Verification items for this drawing (mm, ordinates from the low corner). A direction names the side the tool comes from. Coordinates: 2 decimals unless noted, no trailing zeros. Order: outer loops, then holes, each group sorted by start corner. A loop starts at its lowest first (then second) coordinate and runs counter-clockwise, first axis right, second up.
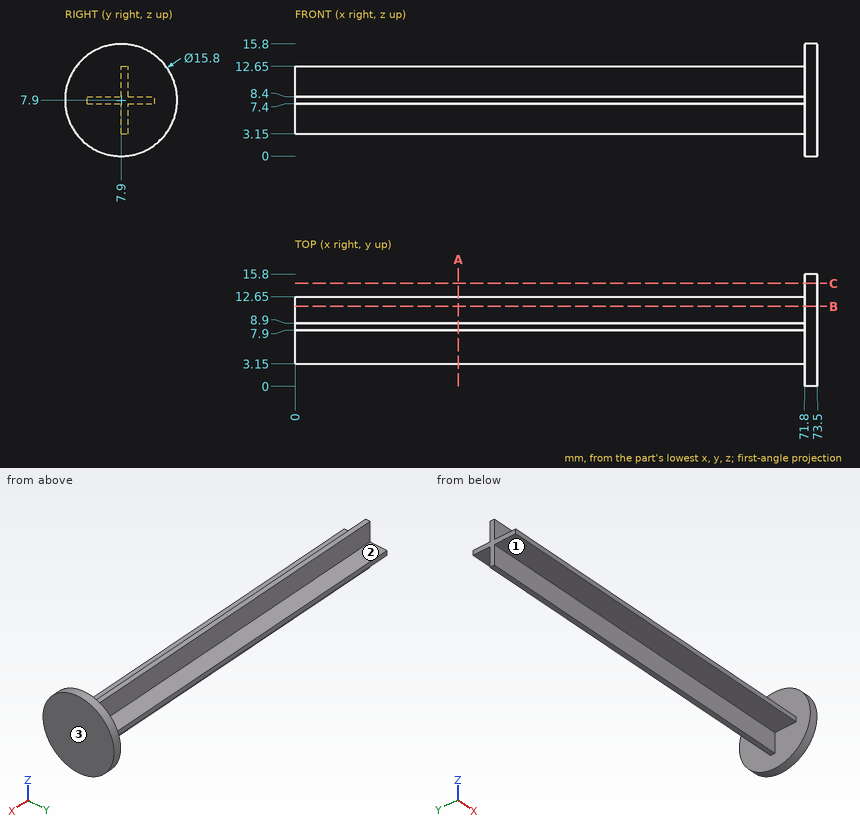
Item 1: Thickness scan on line 1 along X through (y, z) = (3, 2); line 2 along Y through (x, z) = (65.5, 3.5); line 3 along Z through (x, y) = (24.5, 5.25). Record the ranges inside material, lowest first.
Item 2: Depth check by flat-ended pin: P1, Ø4, axis at x = 38, y = 13, coming from the -Z side; P2, Ø5, axis at x = 40.5, y = 5.5, coming from the -Z side; P3, Ø0.5, axis at x = 51.5, y = 8, coming from the +Z side; P4, Ø4.5, axis at y = 8.5, z = 10.5, coming from the -X side. Enter the tip coordinate at first touch or a pass-through.
Item 3: Sectioned sample at B-B (y = 11.25). Record the cut outline in (x, z).
Item 4: Tool access check on the marked faces 1, 2 and 3. Record the directions out of +Z, -Z, +X, -X, +Y, -Y that give a thin tool (end or side, any length) a straight path to the whole face; none if there is none.
Item 5: Sectioned sample at A-A (x = 23). Record the cut outline in (y, z).
Item 6: Sectioned sample at C-C (y = 14.5). Record the cut outline in (x, z), and give its area (3 significant figures).
Geometry check:
1. line 1: x = 71.8 to 73.5
1. line 2: y = 7.9 to 8.9
1. line 3: z = 7.4 to 8.4
2. P1: stops at z = 7.4
2. P2: stops at z = 3.15
2. P3: stops at z = 12.65
2. P4: stops at x = 0
3. outline: (0, 7.4) - (71.8, 7.4) - (71.8, 0.75) - (73.5, 0.75) - (73.5, 15.05) - (71.8, 15.05) - (71.8, 8.4) - (0, 8.4) - close
4. face 1: -Z, -X, -Y
4. face 2: +Z, -X, +Y
4. face 3: +Z, -Z, +X, +Y, -Y
5. outline: (3.15, 7.4) - (7.9, 7.4) - (7.9, 3.15) - (8.9, 3.15) - (8.9, 7.4) - (12.65, 7.4) - (12.65, 8.4) - (8.9, 8.4) - (8.9, 12.65) - (7.9, 12.65) - (7.9, 8.4) - (3.15, 8.4) - close
6. outline: (71.8, 3.56) - (73.5, 3.56) - (73.5, 12.24) - (71.8, 12.24) - close
6. area: 14.8 mm2
